```python
from build123d import *

# Parameters (mm, degrees)
SKETCH2_OUTSIDE_W       = 32.24
SKETCH2_OUTSIDE_H       = 32.24
CUT_EXTRUDE2_DEPTH      = 5.56
SKETCH3_R               = 4.765
CUT_EXTRUDE3_DEPTH      = 14.6
CUT_EXTRUDE4_DEPTH      = 41.799691175
CUT_EXTRUDE4_DEPTH_BACK = 41.799691175
SKETCH4_R               = 1.19


with BuildPart() as part:
    # Sketch1 → Revolve1 (revolve)
    with BuildSketch(Plane.XY, mode=Mode.PRIVATE) as revolve1_sk:
        Polygon((0, 0), (0, 38.1), (6.35, 38.1), (6.35, 21.16), (10.32, 14.06), (10.32, 0), align=None)
    revolve(revolve1_sk.sketch.rotate(Axis((0, 0, 0), (0, 1, 0)), 90), axis=Axis((0, 0, 0), (0, 1, 0)))

    # Sketch2 outside → Cut-Extrude2 (cut)
    with BuildSketch(Plane(origin=(0, 38.1, 0), x_dir=(1, 0, 0), z_dir=(0, 1, 0))):
        Rectangle(SKETCH2_OUTSIDE_W, SKETCH2_OUTSIDE_H)
        with BuildLine():
            Line((4.76, 4.20296324), (4.76, -4.20296324))
            ThreePointArc((4.76, -4.20296324), (-6.35, 0), (4.76, 4.20296324))
        make_face(mode=Mode.SUBTRACT)
    extrude(amount=-CUT_EXTRUDE2_DEPTH, mode=Mode.SUBTRACT)

    # Sketch3 → Cut-Extrude3 (cut)
    with BuildSketch(Plane.XZ):
        with Locations(Location((0, 0, 0), (0, 0, 270))):
            Circle(SKETCH3_R)
    extrude(amount=-CUT_EXTRUDE3_DEPTH, mode=Mode.SUBTRACT)

    # Sketch4 → Cut-Extrude4 (cut, two sides: drawn at the far end of the back side and taken through both)
    with BuildSketch(Plane(origin=(0, 0, 0), x_dir=(0, 0, -1), z_dir=(1, 0, 0)).offset(-CUT_EXTRUDE4_DEPTH_BACK)):
        with Locations((0, 6.35)):
            Circle(SKETCH4_R)
    extrude(amount=CUT_EXTRUDE4_DEPTH + CUT_EXTRUDE4_DEPTH_BACK, mode=Mode.SUBTRACT)


solid = part.part
```
Design review of the part built by this model. Coordinates are the model's own, in mm. A direction names the side the tool comes from. Round coordinates to 2 decimals unless told otherwise and drop trailing zeros. Write each loop counter-clockwise with the first axis right and the second up, starting at its lowest first coordinate (ties: lowest second). Pieces come first, ordered by that corner, then holes.
Item 1: We need section D-D on y = 29.5. Write out the cut boundary in (x, z).
Item 2: We need section A-A on z = 0. Write out the cut boundary in (x, y) (3 decimals).
Item 3: Clearance check with flat-ended pins moving along their axes: pin 1 Ø6 at (y, z) = (35.5, -0.5) entering from +X; pin 2 Ø1 at (x, y) = (-7.5, 15) entering from -Z; pin 3 Ø12 at (x, y) = (6, 15.5) entering from +Z. State where each tip first meets the part, or that it passes through.
Item 4: The part is to be moulded in two halves that separate along Z. For faces 4 (the flat face through (4.76, 35, 0)), 5 (the cylindrical face through (-6.3, 29.5, 0.8)), 6 (the flat face through (0, 14.6, 0)), say which applies: +Z half, -Z half, draft (parallel to the pull), parting line (faces both ways), or undercut.
Item 5: We need section C-C on y = 6.35. Write out the cut boundary in (x, z) (3 decimals), and give its area (3 significant figures).
Item 6: We need section B-B on x = 0. Write out the cut boundary in (y, z) (3 decimals).
Item 7: For faces 1 (the flat face through (-1, 38.1, 0)), 2 (the cylindrical face through (-4.227, 7.198, -2.199)), 3 (the flat face through (5, 32.54, 0)), list the 3-axis set-ups (+Z, -Z, +X, -X, +Y, -Y) from which the entire face can be reached by the end or side of a thin tool; tool diameter is ignored.
Item 8: For probe 1 along Y at (x, z) = (3.5, -2.5); probe 2 along Z at (x, y) = (7.6, 6.35); probe 3 along Z at (x, y) = (8.35, 6.35), list the stretches that pass through material, from the lowest coordinate up.
Returned:
1. outline: circle Ø12.7 at (0, 0)
2. outline: (-10.32, 0) - (-4.765, 0) - (-4.765, 5.16) - (-10.32, 5.16) - close; (-10.32, 7.54) - (-4.765, 7.54) - (-4.765, 14.6) - (4.765, 14.6) - (4.765, 7.54) - (10.32, 7.54) - (10.32, 14.06) - (6.35, 21.16) - (6.35, 32.54) - (4.76, 32.54) - (4.76, 38.1) - (-6.35, 38.1) - (-6.35, 21.16) - (-10.32, 14.06) - close; (4.765, 0) - (10.32, 0) - (10.32, 5.16) - (4.765, 5.16) - close
3. pin 1: stops at x = 6.35
3. pin 2: stops at z = -6.99
3. pin 3: stops at z = 10.32
4. face 4: draft
4. face 5: parting line
4. face 6: undercut
5. outline: (-10.251, -1.19) arc R10.32 ccw to (10.251, -1.19) - (4.614, -1.19) arc R4.765 cw to (-4.614, -1.19) - close; (-10.251, 1.19) - (-4.614, 1.19) arc R4.765 cw to (4.614, 1.19) - (10.251, 1.19) arc R10.32 ccw to start
5. area: 237 mm2
6. outline: (0, -10.32) - (14.06, -10.32) - (21.16, -6.35) - (38.1, -6.35) - (38.1, 6.35) - (21.16, 6.35) - (14.06, 10.32) - (0, 10.32) - (0, 4.765) - (14.6, 4.765) - (14.6, -4.765) - (0, -4.765) - close
7. face 1: +Z, -Z, +X, -X, +Y
7. face 2: -Y
7. face 3: +Z, -Z, +X, +Y
8. probe 1: y = 14.6 to 38.1
8. probe 2: z = -6.98 to -1.19, 1.19 to 6.98
8. probe 3: z = -6.06 to -1.19, 1.19 to 6.06
